Could you check a few things on this drawing? It's one solid part, dimensions in mm from its lowest x, y, z. A direction names the side the tool comes from. Coordinates: 2 decimals unless noted, no trailing zeros. Order: outer loops, then holes, each group sorted by start corner. A loop starts at its lowest first (then second) coordinate and runs counter-clockwise, first axis right, second up. Notation, with made-up numbers: (78, -25) -> (119, -25) arc R20 cw to (119, 0) -> close; hole circle Ø7 at (-27, 52). An arc over 180 degrees is marked (long way). Use a Markdown table: item, result. Add a question column.
1. For the marked faces 4 and 5, which set-ups out of +Z, -Z, +X, -X, +Y, -Y let a thin tool reach every point of the face, with its end or its side?
2. If I drill on line 1 along Y through (x, z) = (25.4, 21); line 2 along Y through (x, z) = (72.5, 20.25) (1 decimal), over which ranges is the centre line in solid material (lowest first)? Write a range as from..to.
3. Suppose I cut it at A-A, the plane z = 9.25. List the corners of the cut face in (x, y) for me.
4. We'd pull the mould along X, two halves only. Please class the marked faces 1, 2 and 3: pulls with the +X half, pulls with the -X half, needs draft (parallel to the pull), parting line crosses it, or undercut.
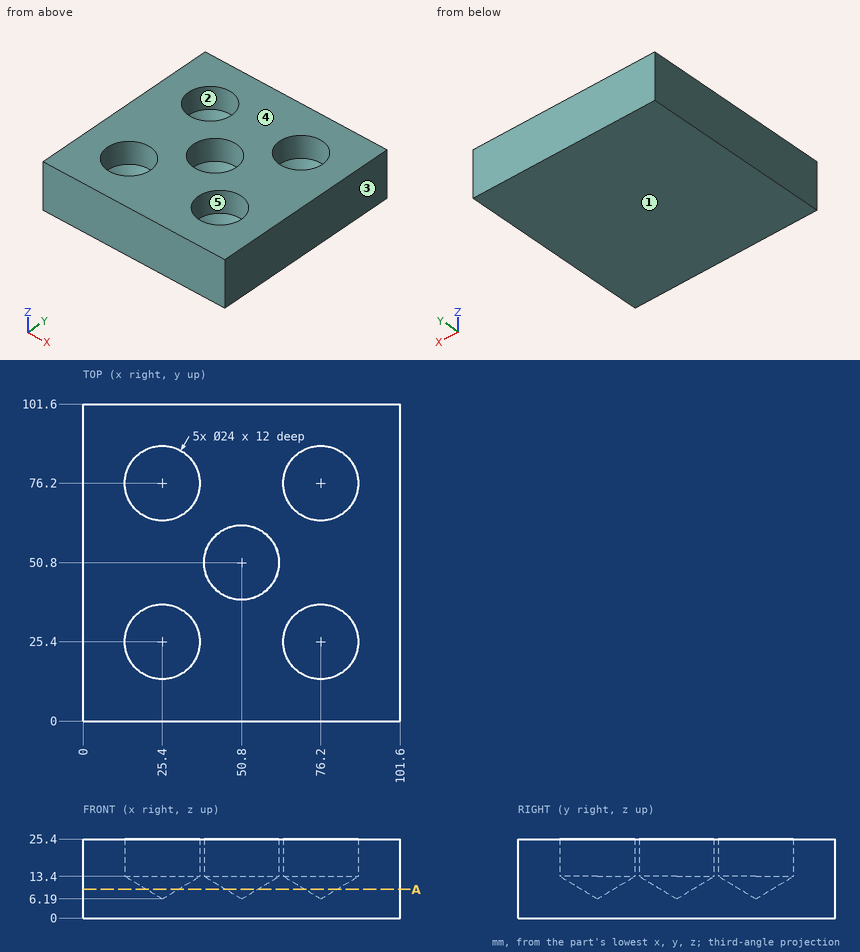
Worked out:
| question | item | result |
|---|---|---|
| 1 | face 4 | +Z, +X, -X, +Y, -Y |
| 1 | face 5 | +Z |
| 2 | line 1 | y = 0..13.4, 37.4..64.2, 88.2..101.6 |
| 2 | line 2 | y = 0..14, 36.8..64.8, 87.6..101.6 |
| 3 | outline | (0, 0) -> (101.6, 0) -> (101.6, 101.6) -> (0, 101.6) -> close; hole circle Ø10.19 at (25.4, 25.4); hole circle Ø10.19 at (25.4, 76.2); hole circle Ø10.19 at (50.8, 50.8); hole circle Ø10.19 at (76.2, 25.4); hole circle Ø10.19 at (76.2, 76.2) |
| 4 | face 1 | needs draft |
| 4 | face 2 | undercut |
| 4 | face 3 | pulls with the +X half |
